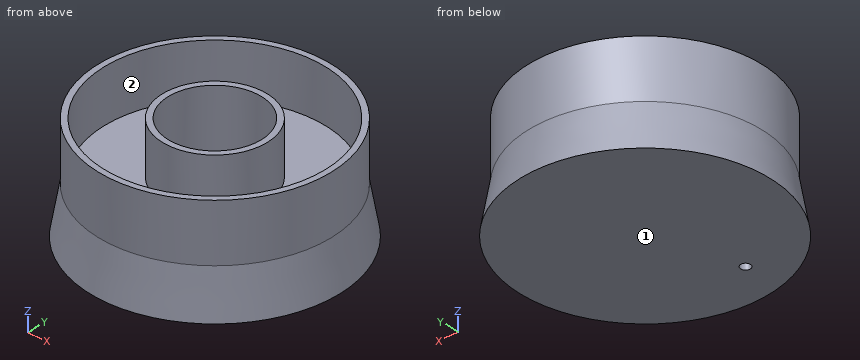
```python
from build123d import *

# Parameters (mm, degrees)
F0_R     = 50
F0_R_2   = 20
F1_DEPTH = 25
F3_T     = -2.5
F4_R     = 50
F5_DEPTH = 20
F5_TAPER = -10
F6_D     = 4.2


with BuildPart() as f1:
    # F0 (on Top) → F1 (new body)
    with BuildSketch(Plane.XY):
        Circle(F0_R)
        Circle(F0_R_2, mode=Mode.SUBTRACT)
    extrude(amount=F1_DEPTH)

    # F3
    f3_openings = [f1.faces().sort_by_distance(p)[0] for p in [
        (-48.585786, 0, 25),
    ]]
    offset(amount=F3_T, openings=f3_openings)

    # F4 (on face) → F5 (join)
    with BuildSketch(Plane(origin=(0, 0, 0), x_dir=(1, 0, 0), z_dir=(0, 0, -1))):
        Circle(F4_R)
    extrude(amount=F5_DEPTH, taper=F5_TAPER)

    # F6 (through all)
    with Locations(Plane.XY.offset(25)):
        with Locations((-12.0698269457, -35.4231074452)):
            Hole(F6_D / 2)


solid = f1.part
```
The listing builds one solid part. Answer for the finished solid, in the listing's coordinates (mm). Face numbers are marked on the shaded views. A direction names the side the tool comes from. Round coordinates to 2 decimals unless told otherwise and drop trailing zeros. Loops run counter-clockwise (first coordinate to the right, second up) from the corner with the lowest first, then second, coordinate; pieces in that order, holes last. Notation, with made-up numbers: (78, 33.5) - (124, 33.5) arc R19 cw to (124, 60.5) - close; hole circle Ø9 at (42.25, 73). An arc over 180 degrees is marked (long way). Use one line per item in the form item = value. Start each with the question number.
1. Given pin 1 Ø8 at (x, z) = (-30.5, -10.5) entering from -Y; pin 2 Ø3 at (x, z) = (-17.5, -8) entering from +Y; pin 3 Ø3 at (y, z) = (29, 3.5) entering from -X; pin 4 Ø2.5 at (x, y) = (-12.07, -35.42) entering from +Z, each flat-ended and moving along its own axis, determine where each tip first touches the part or whether it passes through.
2. The part is cut by section C-C on z = -8.5. Determine the outline of the cut face in (x, y), then the cut area to 3 significant figures.
3. The part is cut by section B-B on x = 0. Determine the outline of the cut face in (y, z).
4. A tool of negligible diameter and unlimited length cuts with its end or side. For the marked faces 1 and 2, from which of +Z, -Z, +X, -X, +Y, -Y can it reach the whole face along a straight path? Write none if from no direction.
5. Consider line 1 (Y direction, x = 0, z = 18.75); line 2 (X direction, y = 10.5, z = 19); line 3 (Y direction, x = 20.5, z = 6). Determine where each line is inside the solid, lowest interval first. Write a range as [from, to].
6. The part is cut by section A-A on z = 16. Determine the outline of the cut face in (x, y).
Geometry check:
q1.pin_1 = -44.71
q1.pin_2 = 48.93
q1.pin_3 = -41.76
q1.pin_4 = through
q2.outline = circle Ø103 at (0, 0); hole circle Ø4.2 at (-12.07, -35.42)
q2.area = 8,320 mm^2
q3.outline = (-53.53, -20) - (53.53, -20) - (50, 0) - (50, 25) - (47.5, 25) - (47.5, 2.5) - (22.5, 2.5) - (22.5, 25) - (20, 25) - (20, 0) - (-20, 0) - (-20, 25) - (-22.5, 25) - (-22.5, 2.5) - (-47.5, 2.5) - (-47.5, 25) - (-50, 25) - (-50, 0) - close
q4.face_1 = -Z, +X, -X, +Y, -Y
q4.face_2 = +Z
q5.line_1 = [-50, -47.5], [-22.5, -20], [20, 22.5], [47.5, 50]
q5.line_2 = [-48.89, -46.32], [-19.9, -17.02], [17.02, 19.9], [46.32, 48.89]
q5.line_3 = [-45.6, -42.85], [-9.27, 9.27], [42.85, 45.6]
q6.outline = circle Ø100 at (0, 0); circle Ø45 at (0, 0); hole circle Ø95 at (0, 0); hole circle Ø40 at (0, 0)
